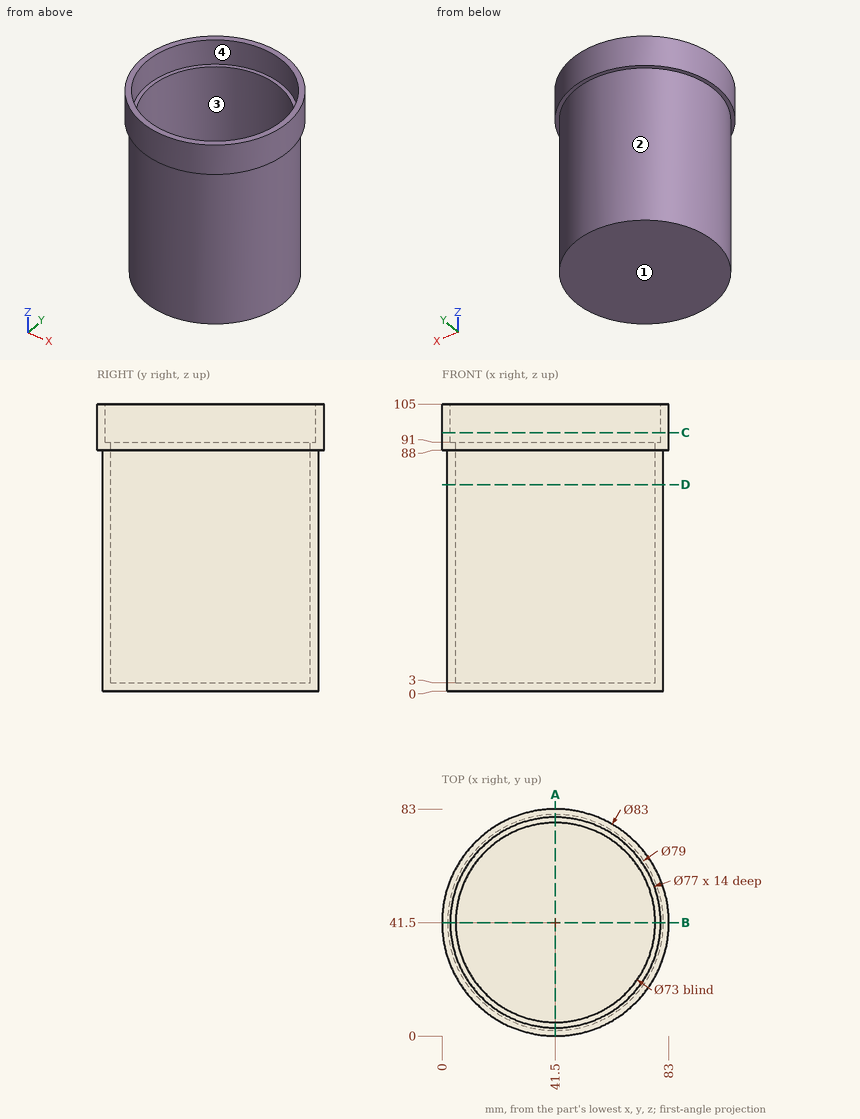
Part print with two shaded views. Sizes in mm from the minimum x, y, z corner. Round coordinates to 2 decimals unless told otherwise and drop trailing zeros. Write each loop counter-clockwise with the first axis right and the second up, starting at its lowest first coordinate (ties: lowest second). Pieces come first, ordered by that corner, then holes. Notation, with made-up numbers: M -39,-6.5 L 4,-6.5 A37 ccw 4,32.5 Z; hole C 48.5,-16 d6. An arc over 180 degrees is marked long. Use CSV: the item, a comma, the result in double quotes.
1. Saw through at D-D (z = 75.5). Give the cut face in (x, y).
Reply:
outline,"C 41.5,41.5 d79; hole C 41.5,41.5 d73"
2. Two-plate mould, pull along X, no slides. Class the marked faces 1, 2, 3 and 4: +X half, -X half, draft (parallel to the pull), parting line (faces both ways), or undercut.
Reply:
face 1,"draft"
face 2,"parting line"
face 3,"undercut"
face 4,"undercut"
3. Wall check: probe 1 along X at (y, z) = (41.5, 97.5); probe 2 along Y at (x, z) = (41.5, 67). Give the ranges that are in metal, low to high. Write a range as from..to.
Reply:
probe 1,"x = 0..3, 80..83"
probe 2,"y = 2..5, 78..81"
4. Flat gauge pins, fed straight in: pin 1 (2 mm diameter, centred on x = 55, z = 44.5, fed in from +Y); pin 2 (12 mm diameter, centred on x = 27.5, z = 21.5, fed in from +Y); pin 3 (12 mm diameter, centred on y = 14.5, z = 33, fed in from -X). Where does each tip first touch, or does it go through?
Reply:
pin 1,"stops at y = 78.97"
pin 2,"stops at y = 80.18"
pin 3,"stops at x = 8.04"
5. Saw through at C-C (z = 94.5). Give the cut face in (x, y).
Reply:
outline,"C 41.5,41.5 d83; hole C 41.5,41.5 d77"
6. Saw through at A-A (x = 41.5). Give the cut face in (y, z), plus the area to 3 significant figures.
Reply:
outline,"M 0,88 L 2,88 L 2,0 L 81,0 L 81,88 L 83,88 L 83,105 L 80,105 L 80,91 L 78,91 L 78,3 L 5,3 L 5,91 L 3,91 L 3,105 L 0,105 Z"
area,"861 mm²"
